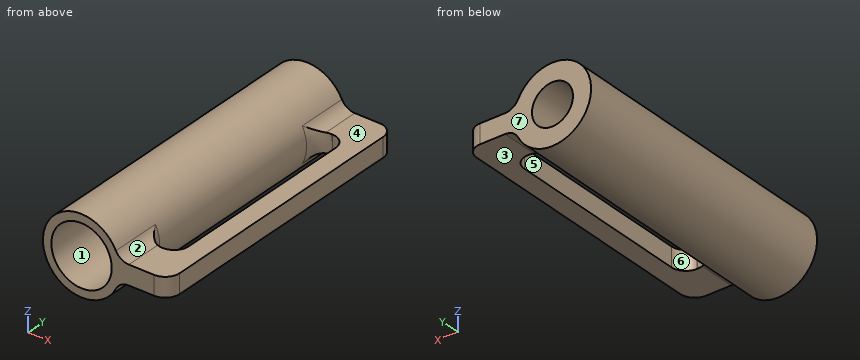
from build123d import *

# Parameters (mm, degrees)
SKETCH1_R           = 8
SKETCH1_R_2         = 4.25
BOSS_EXTRUDE1_DEPTH = 60
BOSS_EXTRUDE2_DEPTH = 2
FILLET1_R           = 3
SKETCH3_R           = 6.25
CUT_EXTRUDE1_DEPTH  = 30


with BuildPart() as part:
    # Sketch1 → Boss-Extrude1 (new body)
    with BuildSketch(Plane(origin=(0, 0, 0), x_dir=(1, 0, 0), z_dir=(0, 1, 0))):
        with Locations(Location((0, 0, 0), (0, 0, 270))):
            Circle(SKETCH1_R)
        with Locations(Location((0, 0, 0), (0, 0, 270))):
            Circle(SKETCH1_R_2, mode=Mode.SUBTRACT)
    extrude(amount=BOSS_EXTRUDE1_DEPTH)

    # Sketch2 → Boss-Extrude2 (add, symmetric)
    with BuildSketch(Plane.XY):
        Polygon((18, 60), (4.25, 60), (4.25, 52.5), (14, 52.5), (14, 7.5), (4.25, 7.5), (4.25, 0), (18, 0), align=None)
    extrude(amount=BOSS_EXTRUDE2_DEPTH, both=True)

    # Fillet1
    fillet1_edges = [part.edges().sort_by_distance(p)[0] for p in [
        (7.745966692, 3.75, -2),
        (7.745966692, 3.75, 2),
        (7.745966692, 56.25, -2),
        (7.745966692, 56.25, 2),
        (18, 0, 0),
        (18, 60, 0),
        (8, 52.5, 0),
        (14, 52.5, 0),
        (8, 7.5, 0),
        (14, 7.5, 0),
    ]]
    fillet(fillet1_edges, radius=FILLET1_R - 0.0001)  # a hair under: the kernel refuses the full size

    # Sketch3 → Cut-Extrude1 (cut)
    with BuildSketch(Plane.XZ):
        with Locations(Location((0, 0, 0), (0, 0, 270))):
            Circle(SKETCH3_R)
    extrude(amount=-CUT_EXTRUDE1_DEPTH, mode=Mode.SUBTRACT)


solid = part.part
Input: part model. Units: mm. Frame: model coordinates. Face numbers are marked on the shaded views. A direction names the side the tool comes from. Give positions to 0.01 mm unless a question says otherwise; leave off trailing zeros. Loops run counter-clockwise (first coordinate to the right, second up) from the corner with the lowest first, then second, coordinate; pieces in that order, holes last. Notation, with made-up numbers: (-16, 88) -> (14, 88) arc R20 ccw to (14, 120) -> close; hole circle Ø4 at (-22.75, 45.25). An arc over 180 degrees is marked (long way). Answer as a JSON object with one key per item and string values. Group by question number.
Item 1: Cut plane B-B, the plane y = 46. Return the cut outline in (x, z).
Item 2: Pull-direction query (Y, two-part tool) for the marked faces 4, 5, 6 and 7; classes: released by +Y, released by -Y, zero draft, split by the parting line, or undercut.
Item 3: Reachability of the marked faces 1, 2 and 3 from +Z, -Z, +X, -X, +Y, -Y: full face, straight path, thin tool, end or side. Return the list, or none.
Item 4: Pin query (flat end, axial travel): P1, Ø4, axis at x = 15.5, y = 17, coming from the -Z side; P2, Ø5, axis at x = 4.5, y = 10, coming from the -Z side; P3, Ø1.2, axis at y = 27, z = -1, coming from the -X side. Return the tip coordinate at first contact, or that it passes through.
Item 5: Cut plane A-A, the plane z = 0. State how many separate pieces and enclosed holes the cut face has, and give its area (3 significant figures).
Item 6: Cut plane C-C, the plane y = 5.5. Return the cut outline in (x, z).
Item 7: Cut plane D-D, the plane x = 0. Return the cut outline in (y, z).
Item 8: Line query: probe 1 along X at (y, z) = (37.5, 0); probe 2 along X at (y, z) = (16, 0); probe 3 along Z at (x, y) = (0, 53.75). Output: solid intervals per line, ascending.
Checks:
{
 "1": {"outline": "circle Ø16 at (0, 0); (14, -2) -> (18, -2) -> (18, 2) -> (14, 2) -> close; hole circle Ø8.5 at (0, 0)"},
 "2": {"face 4": "zero draft", "face 5": "undercut", "face 6": "undercut", "face 7": "released by +Y"},
 "3": {"face 1": "-Y", "face 2": "+Z, +X, +Y, -Y", "face 3": "-Z, +X, +Y, -Y"},
 "4": {"P1": "stops at z = -2", "P2": "stops at z = -7.75", "P3": "stops at x = -7.99"},
 "5": {"separate pieces": "2", "enclosed holes": "1", "area": "664 mm²"},
 "6": {"outline": "(7.13, -3.64) arc R3 cw to (9.8, -2) -> (18, -2) -> (18, 2) -> (9.8, 2) arc R3 cw to (7.13, 3.64) arc R8 ccw (long way) to start; hole circle Ø12.5 at (0, 0)"},
 "7": {"outline": "(0, -8) -> (60, -8) -> (60, -4.25) -> (30, -4.25) -> (30, -6.25) -> (0, -6.25) -> close; (0, 6.25) -> (30, 6.25) -> (30, 4.25) -> (60, 4.25) -> (60, 8) -> (0, 8) -> close"},
 "8": {"probe 1": "x = -8 to -4.25, 4.25 to 8, 14 to 18", "probe 2": "x = -8 to -6.25, 6.25 to 8, 14 to 18", "probe 3": "z = -8 to -4.25, 4.25 to 8"}
}
